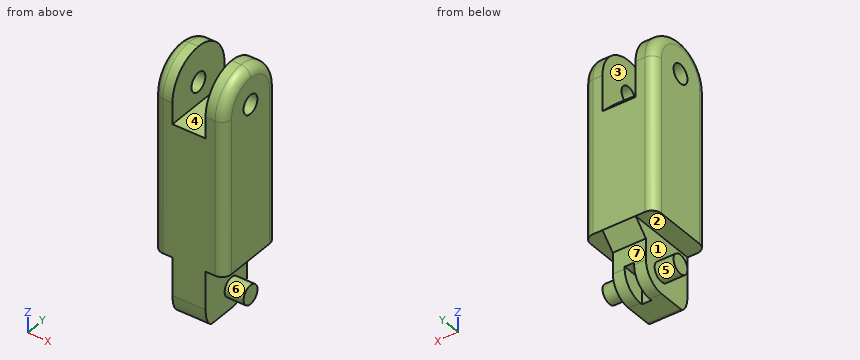
```python
from build123d import *

# Parameters (mm, degrees)
SKETCH1_W                = 15
SKETCH1_H                = 15
BOSS_EXTRUDE1_DEPTH      = 55
SKETCH3_W                = 7
SKETCH3_H                = 15
CUT_EXTRUDE1_DEPTH       = 12
SKETCH4_R                = 2
CUT_EXTRUDE2_DEPTH       = 15
SKETCH5_W                = 4
SKETCH5_H                = 15
CUT_EXTRUDE3_DEPTH       = 15
BOSS_EXTRUDE2_DEPTH      = 7.5
BOSS_EXTRUDE2_DEPTH_BACK = 7.5
SKETCH6_R                = 2
FILLET1_R                = 7.5
CUT_EXTRUDE6_DEPTH       = 3.5
CUT_EXTRUDE6_DEPTH_BACK  = 3.5
FILLET2_R                = 2
CUT_EXTRUDE7_DEPTH       = 7.5
CUT_EXTRUDE7_DEPTH_BACK  = 7.5
FILLET3_SIZE             = 4
FILLET3_SIZE_2           = 2
CUT_EXTRUDE8_DEPTH       = 1
CUT_EXTRUDE8_DEPTH_BACK  = 1


# Some blends are built 0.0001 mm under size
with BuildPart() as part:
    # Sketch1 → Boss-Extrude1 (new body)
    with BuildSketch(Plane.XY):
        Rectangle(SKETCH1_W, SKETCH1_H)
    extrude(amount=BOSS_EXTRUDE1_DEPTH)

    # Sketch3 → Cut-Extrude1 (cut)
    with BuildSketch(Plane.XY.offset(55)):
        Rectangle(SKETCH3_W, SKETCH3_H)
    extrude(amount=-CUT_EXTRUDE1_DEPTH, mode=Mode.SUBTRACT)

    # Sketch4 → Cut-Extrude2 (cut)
    with BuildSketch(Plane(origin=(7.5, 0, 0), x_dir=(0, 0, -1), z_dir=(1, 0, 0))):
        with Locations(Location((-47.5, 0, 0), (0, 0, 90))):
            Circle(SKETCH4_R)
    extrude(amount=-CUT_EXTRUDE2_DEPTH, mode=Mode.SUBTRACT)

    # Sketch5 → Cut-Extrude3 (cut)
    with BuildSketch(Plane(origin=(0, 0, 0), x_dir=(-1, 0, 0), z_dir=(0, 0, -1))):
        with Locations((-5.5, 0)):
            Rectangle(SKETCH5_W, SKETCH5_H)
        with Locations((5.5, 0)):
            Rectangle(SKETCH5_W, SKETCH5_H)
    extrude(amount=-CUT_EXTRUDE3_DEPTH, mode=Mode.SUBTRACT)

    # Sketch6 → Boss-Extrude2 (add, two sides: drawn at the far end of the back side and taken through both)
    with BuildSketch(Plane(origin=(0, 0, 0), x_dir=(0, 0, -1), z_dir=(1, 0, 0)).offset(-BOSS_EXTRUDE2_DEPTH_BACK)):
        with Locations((-7.5, 0)):
            Circle(SKETCH6_R)
    extrude(amount=BOSS_EXTRUDE2_DEPTH + BOSS_EXTRUDE2_DEPTH_BACK)

    # Fillet1
    fillet1_edges = [part.edges().sort_by_distance(p)[0] for p in [
        (5.5, -7.5, 55),
        (-5.5, -7.5, 55),
        (-5.5, 7.5, 55),
        (5.5, 7.5, 55),
    ]]
    fillet(fillet1_edges, radius=FILLET1_R - 0.0001)  # a hair under: the kernel refuses the full size

    # Sketch7 → Cut-Extrude6 (cut, two sides: drawn at the far end of the back side and taken through both)
    with BuildSketch(Plane(origin=(0, 0, 0), x_dir=(0, 0, -1), z_dir=(1, 0, 0)).offset(-CUT_EXTRUDE6_DEPTH_BACK)):
        Polygon((-43, 7.5), (-43, 4.5), (-40, 7.5), align=None)
    extrude(amount=CUT_EXTRUDE6_DEPTH + CUT_EXTRUDE6_DEPTH_BACK, mode=Mode.SUBTRACT)

    # Fillet2
    fillet2_edges = [part.edges().sort_by_distance(p)[0] for p in [
        (7.5, -7.5, 31.25005),
        (7.5, 7.5, 31.25005),
        (7.5, 5.303330148, 52.803330148),
        (7.5, -5.303330148, 52.803330148),
        (-7.5, -7.5, 31.25005),
        (-7.5, 7.5, 31.25005),
        (-7.5, 5.303330148, 52.803330148),
        (-7.5, -5.303330148, 52.803330148),
    ]]
    fillet(fillet2_edges, radius=FILLET2_R)

    # Sketch8 → Cut-Extrude7 (cut, two sides: drawn at the far end of the back side and taken through both)
    with BuildSketch(Plane(origin=(0, 0, 0), x_dir=(0, 0, -1), z_dir=(1, 0, 0)).offset(-CUT_EXTRUDE7_DEPTH_BACK)):
        with BuildLine():
            Line((-15, 7.5), (-12, 4.5))
            Line((-12, 4.5), (-7.5, 4.5))
            ThreePointArc((-7.5, 4.5), (-4.318019485, 3.181980515), (-3, 0))
            Line((-3, 0), (-3, -7.5))
            Line((-3, -7.5), (0, -7.5))
            Line((0, -7.5), (0, 7.5))
            Line((0, 7.5), (-15, 7.5))
        make_face()
    extrude(amount=CUT_EXTRUDE7_DEPTH + CUT_EXTRUDE7_DEPTH_BACK, mode=Mode.SUBTRACT)

    # Fillet3
    # an asymmetric fillet: 4, 2 mm, written as the material it takes off along each edge
    with BuildSketch(Plane(origin=(-13.5, -7.5, 3), x_dir=(0, 0, 1), z_dir=(1, 0, 0))) as fillet3_piece_1:
        with BuildLine():
            Bezier((FILLET3_SIZE, 0), (0, 0), (0, -FILLET3_SIZE_2), weights=[1, 0.707106781, 1])
            Line((0, -FILLET3_SIZE_2), (0, 0))
            Line((0, 0), (FILLET3_SIZE, 0))
        make_face()
    extrude(amount=27, mode=Mode.SUBTRACT)

    # Sketch9 → Cut-Extrude8 (cut, two sides: drawn at the far end of the back side and taken through both)
    with BuildSketch(Plane(origin=(0, 0, 0), x_dir=(0, 0, -1), z_dir=(1, 0, 0)).offset(-CUT_EXTRUDE8_DEPTH_BACK)):
        with BuildLine():
            Line((-8, -0.5), (-8, 9.147620524))
            ThreePointArc((-8, 9.147620524), (-1.178102105, 6.321897895), (1.647620524, -0.5))
            Line((1.647620524, -0.5), (-8, -0.5))
        make_face()
    extrude(amount=CUT_EXTRUDE8_DEPTH + CUT_EXTRUDE8_DEPTH_BACK, mode=Mode.SUBTRACT)


solid = part.part
```
The model under review builds one solid part; all positions refer to its coordinate system, in mm. Face numbers are marked on the shaded views. A direction names the side the tool comes from. Give positions to 0.01 mm unless a question says otherwise; leave off trailing zeros. Write each loop counter-clockwise with the first axis right and the second up, starting at its lowest first coordinate (ties: lowest second). Pieces come first, ordered by that corner, then holes. Notation, with made-up numbers: M 26.5,-30 L 39.5,-30 A19 cw 39.5,-1 Z; hole C 70,18 d2. An arc over 180 degrees is marked long. Write item = value, one per line. Start each with the question number.
Q1. Mouldability with a two-part tool opening along X and no side actions: class the marked faces 1, 2 and 3 as released by +X, released by -X, zero draft, split by the parting line, or undercut.
Q2. For line 1 (Z direction, x = -4.45, y = 0); line 2 (X direction, y = -5.5, z = 49); line 3 (Z direction, x = -6.15, y = 0), list the stretches that pass through material, from the lowest coordinate up.
Q3. Machinability: for the marked faces 4, 5, 6 and 7, which of the approach directions +Z, -Z, +X, -X, +Y, -Y give a long, thin tool a straight path to every point of the face, cutting with its end or side? Answer none if there is none.
Q4. We need section A-A (x = 6.75). Give the number of separate pieces and of enclosed holes in the cut face, plus the area to 3 significant figures.
Q5. We need section B-B (z = 24). State the section outline as (x, y) points.
Q6. Clearance check with flat-ended pins moving along their axes: pin 1 (3 mm diameter, centred on x = 5.5, y = 3, fed in from +Z); pin 2 (7.5 mm diameter, centred on y = 0.5, z = 46.5, fed in from +X); pin 3 (1 mm diameter, centred on x = 5, y = 1.5, fed in from +Z); pin 4 (1.3 mm diameter, centred on x = 1, z = 11, fed in from +Y). State where each tip first meets the part, or that it passes through.
Result set:
q1.face_1 = released by -X
q1.face_2 = zero draft
q1.face_3 = undercut
q2.line_1 = 5.5 to 9.5, 15 to 45.5, 49.5 to 55
q2.line_2 = -7.49 to -3.5, 3.5 to 7.49
q2.line_3 = 5.5 to 9.5, 15 to 45.5, 49.5 to 54.89
q3.face_4 = +Z, +Y, -Y
q3.face_5 = -X
q3.face_6 = +X
q3.face_7 = -Z, +X, -X, +Y
q4.separate_pieces = 2
q4.enclosed_holes = 1
q4.area = 537 mm2
q5.outline = M -7.5,-5.5 A2 ccw -5.5,-7.5 L 5.5,-7.5 A2 ccw 7.5,-5.5 L 7.5,5.5 A2 ccw 5.5,7.5 L -5.5,7.5 A2 ccw -7.5,5.5 Z
q6.pin_1 = 54.85
q6.pin_2 = 7.5
q6.pin_3 = 54.93
q6.pin_4 = 4.5
